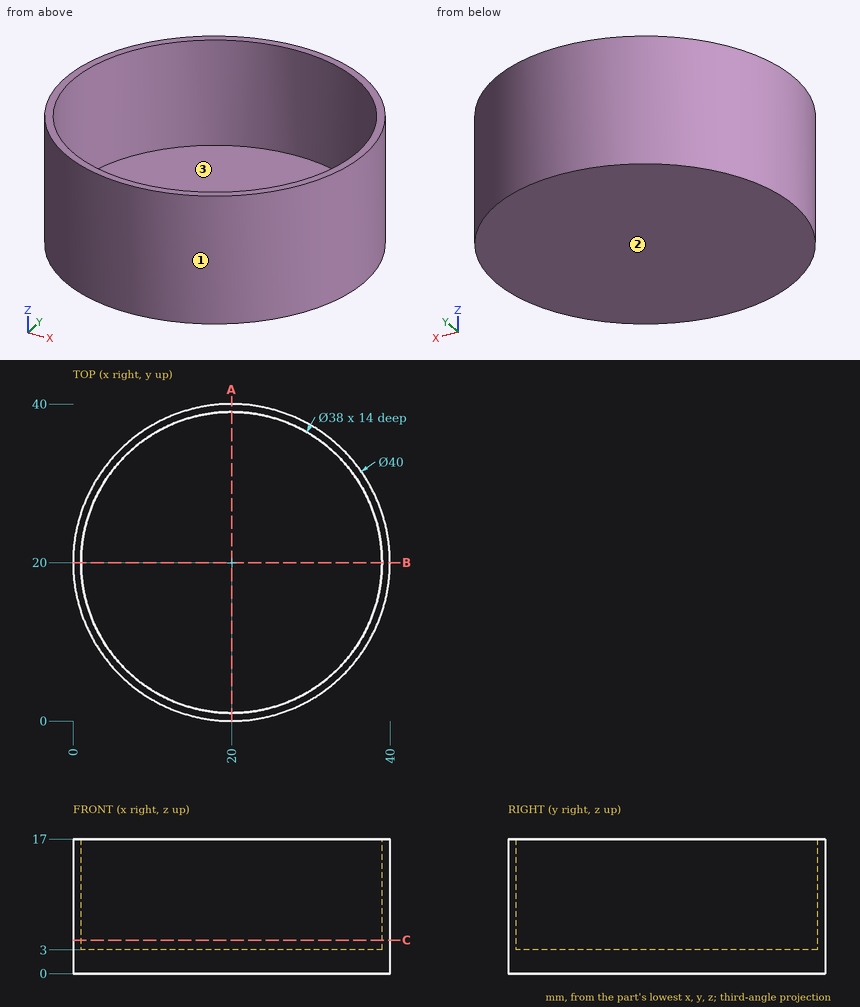
Here's the drawing with two shaded views (mm, measured from the low corner). I have some questions. Coordinates: 2 decimals unless noted, no trailing zeros. Loops run counter-clockwise (first coordinate to the right, second up) from the corner with the lowest first, then second, coordinate; pieces in that order, holes last. Notation, with made-up numbers: (41, 51) -> (79, 51) arc R24 cw to (79, 90) -> close; hole circle Ø1 at (4, 59.25). An arc over 180 degrees is marked (long way). Answer in a Markdown table with one row per item.
(1) Thinking about a two-plate mould opening in Y: for the marked faces 1, 2 and 3, which applies, released by +Y, released by -Y, zero draft, split by the parting line, or undercut?
Results found:
| item | result |
|---|---|
| face 1 | split by the parting line |
| face 2 | zero draft |
| face 3 | undercut |
(2) Imagine slicing it at A-A (x = 20). List the corners of the cut face in (y, z) for me, plus the area to 3 significant figures.
Results found:
| item | result |
|---|---|
| outline | (0, 0) -> (40, 0) -> (40, 17) -> (39, 17) -> (39, 3) -> (1, 3) -> (1, 17) -> (0, 17) -> close |
| area | 148 mm^2 |
(3) Will these pins go through, and if not, where does the flat tip stop? pin 1 Ø1 at (y, z) = (15, 15) entering from +X; pin 2 Ø23 at (x, y) = (20, 20) entering from +Z; pin 3 Ø8 at (x, z) = (15.5, 6) entering from -Y; pin 4 Ø12 at (x, y) = (26, 32.5) entering from -Z.
Results found:
| item | result |
|---|---|
| pin 1 | stops at x = 39.49 |
| pin 2 | stops at z = 3 |
| pin 3 | stops at y = 0.01 |
| pin 4 | stops at z = 0 |
(4) Imagine slicing it at C-C (z = 4.25). List the corners of the cut face in (x, y) for me.
Results found:
| item | result |
|---|---|
| outline | circle Ø40 at (20, 20); hole circle Ø38 at (20, 20) |
(5) If I drill on probe 1 along Y at (x, z) = (20, 14.25); probe 2 along Z at (x, y) = (23.5, 28); probe 3 along Y at (x, z) = (13, 15.75) (3 decimals), over which ranges is the centre line in solid material (lowest first)?
Results found:
| item | result |
|---|---|
| probe 1 | y = 0 to 1, 39 to 40 |
| probe 2 | z = 0 to 3 |
| probe 3 | y = 1.265 to 2.336, 37.664 to 38.735 |
